Autodesk Inventor part; units mm, degrees
ref_plane "YZ Plane" through (0, 0, 0) normal (1, 0, 0) x (0, 1, 0)
ref_plane "XZ Plane" through (0, 0, 0) normal (0, 1, 0) x (-1, 0, 0)
ref_plane "XY Plane" through (0, 0, 0) normal (0, 0, 1) x (1, 0, 0)
sketch "Sketch1" plane through (0, 0, 0) normal (0, 1, 0) x (-1, 0, 0)
  circle A0 centre (0, 0) radius 22.25
  dimension "d0" = 44.5
extrude "Extrusion1" add sketch "Sketch1" along normal blind 8
sketch "Sketch2" plane through (0, 8, 0) normal (0, 1, 0) x (1, 0, 0)
  circle A0 centre (0, 12.7) radius 2.6
  circle A1 centre (0, -12.7) radius 2.6
  point P0 (0, 0)
  dimension "d3" = 5.2
  dimension "d4" = 12.7
  dimension "d5" = 5.2
  dimension "d6" = 12.7
extrude "Extrusion2" cut sketch "Sketch2" against normal up to surface (8 mm away)
sketch "Sketch3" plane through (0, 8, 0) normal (0, 1, 0) x (1, 0, 0)
  circle A0 centre (0, 12.7) radius 2.6
  circle A1 centre (0, 12.7) radius 2.6
  circle A2 centre (0, 12.7) radius 5.6
  point P0 (0, 0)
  dimension "d9" = 3
extrude "Extrusion3" add sketch "Sketch3" along normal blind 5
mirror "Mirror1" about plane through (0, 0, 0) normal (0, 0, 1) of "Extrusion3"
sketch "Sketch4" plane through (0, 0, 0) normal (0, -1, 0) x (1, 0, 0)
  circle A0 centre (0, 0) radius 22.25
  circle A1 centre (0, 0) radius 19.25
  circle A2 centre (0, 0) radius 22.25
  line L0 (2.5, -19.087) -> (-2.5, -19.087) construction
  line L1 (2.5, -19.087) -> (7.5, -19.087) construction
  line L2 (-2.5, -19.087) -> (-4.1056, -21.8679)
  line L3 (-2.5, -19.087) -> (0.7112, -19.087) construction
  line L4 (2.5, -19.087) -> (4.1056, -21.8679)
  line L5 (2.5, -19.087) -> (5.7112, -19.087) construction
  point P0 (4.1056, -21.8679)
  point P1 (-4.1056, -21.8679)
  dimension "d17" = 3
  dimension "d18" = 5
  dimension "d19" = 180
  dimension "d20" = 120
  dimension "d21" = 60
extrude "Extrusion5" add sketch "Sketch4" along normal blind 11 contours L2 A1 L4 A0 picked at (0.2785, -21.2156)
pattern_circular "Circular Pattern1" count 12 over 360 about axis through (0, -10, 0) along (0, 1, 0) of "Extrusion5"
fillet "Fillet1" radius 3 2 edges at (-5.6, 13, -12.7) (-5.6, 13, 12.7)
sketch "Sketch6" plane through (0, 8, 0) normal (0, 1, 0) x (1, 0, 0)
  circle A0 centre (0, 0) radius 22.25
  circle A1 centre (0, 0) radius 22.25
  line L0 (7, 9) -> (7, -9)
  line L1 (7, 9) -> (25, 9) construction
  line L2 (7, 9) -> (20.3485, 9)
  line L3 (7, -9) -> (20.3485, -9)
  point P0 (7, 0)
  dimension "d29" = 18
  dimension "d30" = 90
  dimension "d56" = 7
extrude "Extrusion6" cut sketch "Sketch6" against normal blind 7 contours A0 L3 L0 L2 picked at (12.0833, 0)
sketch "Sketch7" plane through (0, 8, 0) normal (0, 1, 0) x (1, 0, 0)
  circle A0 centre (0, 0) radius 19.25 construction
  arc A1 (20.3485, 9) -> (20.3485, -9) centre (0, 0) ccw construction
  circle A2 centre (3, 7) radius 2.5
  arc A3 (4.1056, 21.8679) -> (-4.1056, 21.8679) centre (0, 0) ccw construction
  line L0 (0, 22.25) -> (0, -22.25) construction
  arc A4 (-4.1056, -21.8679) -> (4.1056, -21.8679) centre (0, 0) ccw construction
  line L1 (22.25, 0) -> (-22.25, 0) construction
  arc A5 (-21.8679, 4.1056) -> (-21.8679, -4.1056) centre (0, 0) ccw construction
  line L2 (7, -9) -> (7, 9) construction
  circle A6 centre (3, 0) radius 2.5
  circle A7 centre (3, -7) radius 2.5
  circle A8 centre (0, 0) radius 5.5
  circle A9 centre (-18, 7) radius 2.5
  circle A10 centre (-18, 0) radius 2.5
  circle A11 centre (-18, -7) radius 2.5
  dimension "d34" = 3
  dimension "d35" = 5
  dimension "d36" = 4
  dimension "d39" = 7
  dimension "d44" = 11
  dimension "d45" = 5
  dimension "d48" = 7
  dimension "d53" = 21
extrude "Extrusion7" cut sketch "Sketch7" against normal up to surface (8 mm away) contours A8 A2 | A6 | A2 A8 A7 | A7 A8 | A9 | A10 | A11 picked at (2.1127, 4.9296) picked at (2.1127, -4.9296)
sketch "Sketch9" plane through (0, 1, 0) normal (0, 1, 0) x (1, 0, 0)
  line L0 (7, -9) -> (7, 9)
  line L1 (20.3485, -9) -> (7, -9)
  line L2 (7, 9) -> (18.9991, 9)
  line L3 (18.9991, 9) -> (18.9991, -9)
  line L4 (18.9991, -9) -> (7, -9)
  line L5 (7, -9) -> (7, 9)
  point P0 (0, 0)
extrude "Extrusion8" cut sketch "Sketch9" against normal through all
equation "\"d5\" = d3"
equation "\"d34\" = d17"
equation "\"d45\" = d35"
properties part number "spacer"
Geometry: final body of the model. Coordinates: model frame, mm. A direction names the side the tool comes from. Round coordinates to 2 decimals unless told otherwise and drop trailing zeros. Loops run counter-clockwise (first coordinate to the right, second up) from the corner with the lowest first, then second, coordinate; pieces in that order, holes last.
Q1. Material intervals for L1, parallel to Z at x = 0, y = 7.25; L2, parallel to X at y = 3.25, z = 0.5; L3, parallel to Z at x = -18, y = 2.25, sorted ascending.
Q2. Access query for faces 5 (the flat face through (-10, -11, -18)), 6 (the cylindrical face through (-0.338, 6.409, 15.278)), 7 (the flat face through (-16.07, -5.42, 13.08)), 8 (the flat face through (-6, 0, 0)), 9 (the cylindrical face through (-20.5, 4.1, -0.1)). Directions: +Z, -Z, +X, -X, +Y, -Y. A direction counts if a zero-diameter tool reaches every point of the face in a straight line with its end or side. Return the directions, or none.
Q3. Pull-direction query (Z, two-part tool) for faces 1 (the cylindrical face through (-0.04, -5.42, 19.25)), 2 (the flat face through (20, 1, 0)), 3 (the flat face through (-16.07, -5.42, -13.08)), 4 (the flat face through (0, -11, -21)); classes: released by +Z, released by -Z, zero draft, split by the parting line, or undercut.
Q4. Section A-A on z = 0. Return loops of the section in (x, y), plus the area to 3 significant figures.
Q5. Pin query (flat end, axial travel): P1, Ø8, axis at y = -7.5, z = -16, coming from the -X side; P2, Ø6, axis at y = -3.5, z = 8.5, coming from the +X side; P3, Ø0.6, axis at x = -19.5, z = -8.5, coming from the +Y side; P4, Ø12, axis at x = 12.5, z = -12.5, coming from the -Y side. Return the tip coordinate at first contact, or that it passes through.
Q6. Section B-B on x = 0. State how many separate pieces and enclosed holes the cut face has, plus the area to 3 significant figures.
Evaluation:
1. L1: z = -22.25 to -15.3, -10.1 to -5.5, 5.5 to 10.1, 15.3 to 22.25
1. L2: x = -22.24 to -20.45, -15.55 to -5.48, 5.48 to 7
1. L3: z = -13.08 to -9.5, -4.5 to -2.5, 2.5 to 4.5, 9.5 to 13.08
2. face 5: +Z, -Z, +X, -X, -Y
2. face 6: +Y, -Y
2. face 7: +Z, -Y
2. face 8: -Y
2. face 9: +Y
3. face 1: undercut
3. face 2: undercut
3. face 3: released by -Z
3. face 4: zero draft
4. outline: (-22.25, -11) - (-19.25, -11) - (-19.25, 0) - (-20.5, 0) - (-20.5, 8) - (-22.25, 8) - close; (-15.5, 0) - (-5.5, 0) - (-5.5, 8) - (-15.5, 8) - close; (5.5, 0) - (7, 0) - (7, 8) - (5.5, 8) - close; (19, 0) - (19.25, 0) - (19.25, -11) - (22.25, -11) - (22.25, 1) - (19, 1) - close
4. area: 175 mm2
5. P1: stops at x = -18.74
5. P2: stops at x = 20.99
5. P3: stops at y = 0
5. P4: stops at y = -11
6. separate pieces: 4
6. enclosed holes: 0
6. area: 303 mm2
